Verification items for the finished model (mm, model axes). A direction names the side the tool comes from. Coordinates: 2 decimals unless noted, no trailing zeros. Write each loop counter-clockwise with the first axis right and the second up, starting at its lowest first coordinate (ties: lowest second). Pieces come first, ordered by that corner, then holes. Notation, with made-up numbers: (89.25, 20.5) -> (142.25, 20.5) arc R27 cw to (142.25, 51.5) -> close; hole circle Ø5 at (56.5, -30.75). An arc over 180 degrees is marked (long way). Use CSV: the item, a comma, the result in double quotes.
Autodesk Fusion 360 part; units mm, degrees
sketch "Boceto1" plane through (0, 0, 0) normal (1, 0, 0) x (0, 1, 0)
  circle A0 centre (0, 0) radius 25
  dimension "d1" = 50
extrude "Wheel width" add sketch "Boceto1" along normal blind 26
sketch "Boceto2" plane through (26, 0, 0) normal (1, 0, 0) x (0, 1, 0)
  circle A0 centre (0, 0) radius 25
  circle A1 centre (0, 0) radius 5
  circle A2 centre (0, 0) radius 9
  dimension "d4" = 10
  dimension "d5" = 18
extrude "Wheel profile 1 (1)" cut sketch "Boceto2" against normal blind 3 contours A2
sketch "Boceto3" plane through (26, 0, 0) normal (1, 0, 0) x (0, 1, 0)
  circle A0 centre (0, 0) radius 25
  circle A1 centre (0, 0) radius 9
  circle A2 centre (0, 0) radius 23.5
  line L0 (0, 23.5) -> (0, 13.5) construction
  line L1 (0, 13.5) -> (-5, 13.5)
  line L2 (0, 13.5) -> (5, 13.5)
  line L3 (0, 23.5) -> (-2.5, 23.5)
  line L4 (-2.5, 23.5) -> (-5, 13.5)
  line L5 (2.5, 23.5) -> (5, 13.5)
  line L6 (0, 23.5) -> (2.5, 23.5)
  line L7 (-12.8393, 4.1717) -> (-11.2942, 8.927)
  line L8 (-12.8393, 4.1717) -> (-14.3843, -0.5836)
  line L9 (-23.1224, 4.8843) -> (-14.3843, -0.5836)
  line L10 (-22.3498, 7.2619) -> (-23.1224, 4.8843)
  line L11 (-22.3498, 7.2619) -> (-21.5773, 9.6395)
  line L12 (-21.5773, 9.6395) -> (-11.2942, 8.927)
  line L13 (-7.9351, -10.9217) -> (-11.9802, -7.9828)
  line L14 (-7.9351, -10.9217) -> (-3.89, -13.8607)
  line L15 (-11.7904, -20.4814) -> (-3.89, -13.8607)
  line L16 (-13.813, -19.0119) -> (-11.7904, -20.4814)
  line L17 (-13.813, -19.0119) -> (-15.8355, -17.5424)
  line L18 (-15.8355, -17.5424) -> (-11.9802, -7.9828)
  line L19 (7.9351, -10.9217) -> (3.89, -13.8607)
  line L20 (7.9351, -10.9217) -> (11.9802, -7.9828)
  line L21 (15.8355, -17.5424) -> (11.9802, -7.9828)
  line L22 (13.813, -19.0119) -> (15.8355, -17.5424)
  line L23 (13.813, -19.0119) -> (11.7904, -20.4814)
  line L24 (11.7904, -20.4814) -> (3.89, -13.8607)
  line L25 (12.8393, 4.1717) -> (14.3843, -0.5836)
  line L26 (12.8393, 4.1717) -> (11.2942, 8.927)
  line L27 (21.5773, 9.6395) -> (11.2942, 8.927)
  line L28 (22.3498, 7.2619) -> (21.5773, 9.6395)
  line L29 (22.3498, 7.2619) -> (23.1224, 4.8843)
  line L30 (23.1224, 4.8843) -> (14.3843, -0.5836)
  arc A3 (-11.2942, 8.927) -> (-5, 13.5) centre (-10.8755, 14.9689) ccw
  arc A4 (-11.9802, -7.9828) -> (-14.3843, -0.5836) centre (-17.597, -5.7176) ccw
  arc A5 (3.89, -13.8607) -> (-3.89, -13.8607) centre (0, -18.5026) ccw
  arc A6 (14.3843, -0.5836) -> (11.9802, -7.9828) centre (17.597, -5.7176) ccw
  arc A7 (5, 13.5) -> (11.2942, 8.927) centre (10.8755, 14.9689) ccw
  dimension "d8" = 47
  dimension "d9" = 10
  dimension "d10" = 5
  dimension "d12" = 2.5
  dimension "d14" = 360
extrude "Wheel profile 2 (1)" cut sketch "Boceto3" against normal through all contours A2 L21 L30 A6 | A2 L5 L27 A7 | A2 L15 L24 A5 | A2 L4 L12 A3 | A2 L9 L18 A4
sketch "Boceto4" plane through (0, 0, 0) normal (-1, 0, 0) x (0, -1, 0)
  line L0 (-11.9802, -7.9828) -> (-15.7827, -17.4114)
  arc A0 (-23.0026, 4.8093) -> (-15.7827, -17.4114) centre (0, 0) ccw
  line L1 (-23.0026, 4.8093) -> (-14.3843, -0.5836)
  arc A1 (-11.9802, -7.9828) -> (-14.3843, -0.5836) centre (-17.597, -5.7176) ccw
  line L2 (-11.2942, 8.927) -> (-21.4364, 9.6298)
  arc A2 (-2.5343, 23.363) -> (-21.4364, 9.6298) centre (0, 0) ccw
  line L3 (-2.5343, 23.363) -> (-5, 13.5)
  arc A3 (-11.2942, 8.927) -> (-5, 13.5) centre (-10.8755, 14.9689) ccw
  line L4 (3.89, -13.8607) -> (11.6821, -20.3906)
  arc A4 (-11.6821, -20.3906) -> (11.6821, -20.3906) centre (0, 0) ccw
  line L5 (-11.6821, -20.3906) -> (-3.89, -13.8607)
  arc A5 (3.89, -13.8607) -> (-3.89, -13.8607) centre (0, -18.5026) ccw
  line L6 (5, 13.5) -> (2.5343, 23.363)
  arc A6 (21.4364, 9.6298) -> (2.5343, 23.363) centre (0, 0) ccw
  line L7 (21.4364, 9.6298) -> (11.2942, 8.927)
  arc A7 (5, 13.5) -> (11.2942, 8.927) centre (10.8755, 14.9689) ccw
  line L8 (14.3843, -0.5836) -> (23.0026, 4.8093)
  arc A8 (15.7827, -17.4114) -> (23.0026, 4.8093) centre (0, 0) ccw
  line L9 (15.7827, -17.4114) -> (11.9802, -7.9828)
  arc A9 (14.3843, -0.5836) -> (11.9802, -7.9828) centre (17.597, -5.7176) ccw
  circle A10 centre (0, 0) radius 25
  circle A11 centre (0, 0) radius 23.5
extrude "Wheel hole (1)" cut sketch "Boceto4" against normal blind 21 contours L0 L1 A1 L2 L3 A3 L4 L5 A5 L6 L7 A7 L8 L9 A9 A11
sketch "Boceto5" plane through (21, 0, 0) normal (-1, 0, 0) x (0, -1, 0)
  line L0 (3.89, -13.8607) -> (11.6821, -20.3906)
  arc A0 (11.6821, -20.3906) -> (15.7827, -17.4114) centre (0, 0) ccw
  line L1 (15.7827, -17.4114) -> (11.9802, -7.9828)
  arc A1 (14.3843, -0.5836) -> (11.9802, -7.9828) centre (17.597, -5.7176) ccw
  line L2 (14.3843, -0.5836) -> (23.0026, 4.8093)
  arc A2 (23.0026, 4.8093) -> (21.4364, 9.6298) centre (0, 0) ccw
  line L3 (21.4364, 9.6298) -> (11.2942, 8.927)
  arc A3 (5, 13.5) -> (11.2942, 8.927) centre (10.8755, 14.9689) ccw
  line L4 (5, 13.5) -> (2.5343, 23.363)
  arc A4 (2.5343, 23.363) -> (-2.5343, 23.363) centre (0, 0) ccw
  line L5 (-2.5343, 23.363) -> (-5, 13.5)
  arc A5 (-11.2942, 8.927) -> (-5, 13.5) centre (-10.8755, 14.9689) ccw
  line L6 (-11.2942, 8.927) -> (-21.4364, 9.6298)
  arc A6 (-21.4364, 9.6298) -> (-23.0026, 4.8093) centre (0, 0) ccw
  line L7 (-23.0026, 4.8093) -> (-14.3843, -0.5836)
  arc A7 (-11.9802, -7.9828) -> (-14.3843, -0.5836) centre (-17.597, -5.7176) ccw
  line L8 (-11.9802, -7.9828) -> (-15.7827, -17.4114)
  arc A8 (-15.7827, -17.4114) -> (-11.6821, -20.3906) centre (0, 0) ccw
  line L9 (-11.6821, -20.3906) -> (-3.89, -13.8607)
  arc A9 (3.89, -13.8607) -> (-3.89, -13.8607) centre (0, -18.5026) ccw
  circle A10 centre (0, 0) radius 5
  dimension "d18" = 10
extrude "Connector base (1)" add sketch "Boceto5" along normal blind 10 contours A10
sketch "Boceto6" plane through (11, 0, 0) normal (-1, 0, 0) x (0, -1, 0)
  circle A0 centre (0, 0) radius 5
  line L0 (1.85, 1.9666) -> (-1.85, 1.9666)
  line L1 (-1.85, -1.9666) -> (1.85, -1.9666)
  arc A1 (-1.85, 1.9666) -> (-1.85, -1.9666) centre (0, 0) ccw
  arc A2 (1.85, -1.9666) -> (1.85, 1.9666) centre (0, 0) ccw
  dimension "d21" = 5.4
  dimension "d22" = 3.7
extrude "Connector hole (1)" cut sketch "Boceto6" against normal blind 9 contours L0 L1 A1 A2
1) Mould release check, pull along Y, two halves, no side actions. Record for faces 1 (the flat face through (0, -17, -17)), 2 (the cylindrical face through (12.818, 23.846, -7.509)), 3 (the cylindrical face through (23.535, 11.856, -3.79)): released by +Y, released by -Y, zero draft, split by the parting line, or undercut.
Return value:
face 1,"zero draft"
face 2,"split by the parting line"
face 3,"undercut"
2) Gauge pin test, flat ends, axial feed: pin 1 (3 mm diameter, centred on y = 0, z = 13, fed in from -X); pin 2 (1.8 mm diameter, centred on x = 13.5, y = 0, fed in from -Z); pin 3 (1.2 mm diameter, centred on y = 1, z = 0, fed in from -X). Record the tip position at first contact, or that the pin passes through.
Return value:
pin 1,"x = 21"
pin 2,"z = -25"
pin 3,"x = 20"
3) Cross-section at B-B (y = 0). Record the boundary of the cut face in (x, z).
Return value:
outline,"(0, -25) -> (26, -25) -> (26, -23.5) -> (0, -23.5) -> close; (0, 23.5) -> (21, 23.5) -> (21, 5) -> (11, 5) -> (11, 1.97) -> (20, 1.97) -> (20, -1.97) -> (11, -1.97) -> (11, -5) -> (21, -5) -> (21, -12.45) -> (26, -12.45) -> (26, -9) -> (23, -9) -> (23, -5) -> (26, -5) -> (26, 5) -> (23, 5) -> (23, 9) -> (26, 9) -> (26, 25) -> (0, 25) -> close"
4) Scan lines: L1, parallel to Z at x = 23.6, y = 0; L2, parallel to Z at x = 17.5, y = 0; L3, parallel to Y at x = 22, z = 3. Record each from-to range of solid material in increasing order.
Return value:
L1,"-25 to -23.5, -12.45 to -9, -5 to 5, 9 to 25"
L2,"-25 to -23.5, -5 to -1.97, 1.97 to 5, 23.5 to 25"
L3,"-24.82 to -23.31, -20.11 to 20.11, 23.31 to 24.82"
5) Cross-section at A-A (x = 16.5). Record the boundary of the cut face in (y, z), plus the area to 3 significant figures.
Return value:
outline,"circle Ø50 at (0, 0); circle Ø10 at (0, 0); hole circle Ø47 at (0, 0); hole (-1.85, -1.97) -> (1.85, -1.97) arc R2.7 ccw to (1.85, 1.97) -> (-1.85, 1.97) arc R2.7 ccw to start"
area,"288 mm2"
6) Set-up check for faces 4 (the cylindrical face through (16.07, 1.08, 4.88)), 5 (the cylindrical face through (23.54, -11.82, -3.9)), 6 (the cylindrical face through (24.52, -1.08, -4.88)), 7 (the flat face through (26, 0, 0)): record each of +Z, -Z, +X, -X, +Y, -Y from which the full face is reachable in a straight line by a thin tool's end or side.
Return value:
face 4,"-X"
face 5,"+X, -X"
face 6,"+X"
face 7,"+Z, -Z, +X, +Y, -Y"
7) Cross-section at C-C (y = 10). Record the boundary of the cut face in (x, z).
Return value:
outline,"(0, -22.91) -> (26, -22.91) -> (26, -21.27) -> (0, -21.27) -> close; (0, 21.27) -> (26, 21.27) -> (26, 22.91) -> (0, 22.91) -> close; (21, -18.98) -> (26, -18.98) -> (26, 8.98) -> (21, 8.98) -> close"
8) Cross-section at D-D (x = 21.75). Record the boundary of the cut face in (y, z).
Return value:
outline,"circle Ø50 at (0, 0); hole (-23, 4.81) arc R23.5 ccw to (-15.78, -17.41) -> (-11.98, -7.98) arc R6.06 ccw to (-14.38, -0.58) -> close; hole (-21.44, 9.63) -> (-11.29, 8.93) arc R6.06 ccw to (-5, 13.5) -> (-2.53, 23.36) arc R23.5 ccw to start; hole (-11.68, -20.39) arc R23.5 ccw to (11.68, -20.39) -> (3.89, -13.86) arc R6.06 ccw to (-3.89, -13.86) -> close; hole (2.53, 23.36) -> (5, 13.5) arc R6.06 ccw to (11.29, 8.93) -> (21.44, 9.63) arc R23.5 ccw to start; hole (11.98, -7.98) -> (15.78, -17.41) arc R23.5 ccw to (23, 4.81) -> (14.38, -0.58) arc R6.06 ccw to start"
